For this review, take the finished solid that the model builds, in its own axes (mm). Face numbers are marked on the shaded views. A direction names the side the tool comes from. Coordinates: 2 decimals unless noted, no trailing zeros. Loops run counter-clockwise (first coordinate to the right, second up) from the corner with the lowest first, then second, coordinate; pieces in that order, holes last. Notation, with made-up numbers: (-15.5, -8) - (22.5, -8) arc R11 ccw to (22.5, 12) - close; hole circle Ø9 at (13, 33). An arc over 180 degrees is marked (long way). Use one line per item in the form item = value. Start each with the question number.
1. Machinability: for the marked faces 1 and 2, which of the approach directions +Z, -Z, +X, -X, +Y, -Y give a long, thin tool a straight path to every point of the face, cutting with its end or side? Answer none if there is none.
2. Add section C-C on z = 219. Give the boundary of the cut face in (x, y), and give its area (3 significant figures).
3. For pin 1 Ø1 at (x, z) = (182, 177) entering from +Y; pin 2 Ø24 at (y, z) = (-21, 23) entering from +X; pin 3 Ø7.5 at (x, y) = (286, -23.5) entering from -Z, all flat-tipped, find the tip position at first contact; note any pin that passes through.
4. Add section D-D on y = 488. Give the boundary of the cut face in (x, z), and give its area (4 significant figures).
5. Add section B-B on x = 114. Give the boundary of the cut face in (y, z), and give its area (3 significant figures).
6. To check wall thickness, follow probe 1 along Y at (x, z) = (-208, 682); probe 2 along Z at (x, y) = (-15.5, 1068.5). State the ranges of each line that lie inside material, in increasing order.
7. Add section A-A on y = 24.5. Give the boundary of the cut face in (x, z).
```python
from build123d import *

# Parameters (mm, degrees)
F0_W     = 600
F0_H     = 100
F1_DEPTH = 800
F2_W     = 100
F2_H     = 80
F3_DEPTH = 25
F4_W     = 630
F4_H     = 100
F5_DEPTH = 25
F6_W     = 630
F6_H     = 25
F7_DEPTH = 1100


with BuildPart() as f1:
    # F0 (on Top) → F1 (new body)
    with BuildSketch(Plane.XY):
        Rectangle(F0_W, F0_H)
    extrude(amount=F1_DEPTH)

    # F2 (on face) → F3 (cut)
    with BuildSketch(Plane.YZ.offset(300)):
        with Locations((0, 40)):
            Rectangle(F2_W, F2_H)
    extrude(amount=-F3_DEPTH, mode=Mode.SUBTRACT)

    # F4 (on face) → F5 (join)
    with BuildSketch(Plane.XY.offset(800)):
        with Locations((15, 0)):
            Rectangle(F4_W, F4_H)
    extrude(amount=F5_DEPTH)

    # F6 (on face) → F7 (join)
    with BuildSketch(Plane(origin=(0, 50, 0), x_dir=(-1, 0, 0), z_dir=(0, 1, 0))):
        with Locations((-15, 812.5)):
            Rectangle(F6_W, F6_H)
    extrude(amount=F7_DEPTH)


solid = f1.part
```
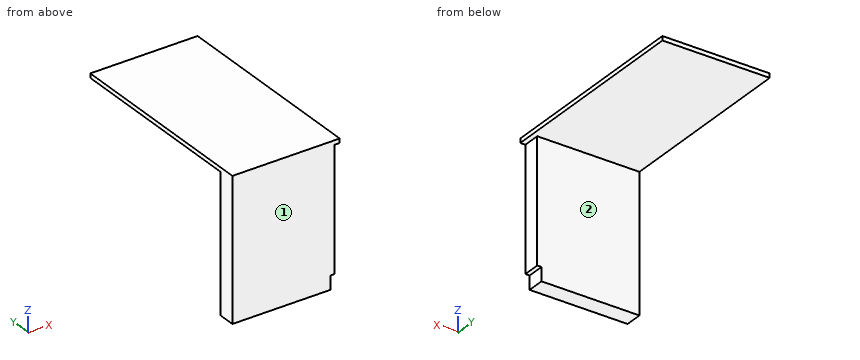
Conclusion:
q1.face_1 = +Z, -Z, +X, -X, -Y
q1.face_2 = -Z, +X, -X, +Y
q2.outline = (-300, -50) - (300, -50) - (300, 50) - (-300, 50) - close
q2.area = 60,000 mm^2
q3.pin_1 = 50
q3.pin_2 = 275
q3.pin_3 = 80
q4.outline = (-300, 800) - (330, 800) - (330, 825) - (-300, 825) - close
q4.area = 15,750 mm^2
q5.outline = (-50, 0) - (50, 0) - (50, 800) - (1150, 800) - (1150, 825) - (-50, 825) - close
q5.area = 110,000 mm^2
q6.probe_1 = -50 to 50
q6.probe_2 = 800 to 825
q7.outline = (-300, 0) - (275, 0) - (275, 80) - (300, 80) - (300, 800) - (330, 800) - (330, 825) - (-300, 825) - close
